Check sheet for the modelled part. Datum: model origin and axes. Units: mm. Face numbers are marked on the shaded views. A direction names the side the tool comes from. Round coordinates to 2 decimals unless told otherwise and drop trailing zeros. Write each loop counter-clockwise with the first axis right and the second up, starting at its lowest first coordinate (ties: lowest second). Pieces come first, ordered by that corner, then holes. Notation, with made-up numbers: (-14.75, 20) -> (27.25, 20) arc R33 ccw to (27.25, 57) -> close; hole circle Ø9 at (-25.5, 76.5). An arc over 180 degrees is marked (long way). One line per item, written item: value.
from build123d import *

# Parameters (mm, degrees)
SKETCH_1_R          = 1.25
SKETCH_1_R_2        = 1.5
EXTRUDE_1_DEPTH     = 0.5
SKETCH_2_W          = 9
SKETCH_2_H          = 0.5
EXTRUDE_2_DEPTH     = 5
CUT_EXTRUDE_1_REACH = 16.195
SKETCH_3_R          = 1


with BuildPart() as part:
    # 草图1 → 凸台-拉伸1 (new body)
    with BuildSketch(Plane.XY):
        with BuildLine():
            Line((0, 0), (9, 0))
            Line((9, 0), (6.667108595, 8.355095313))
            ThreePointArc((6.667108595, 8.355095313), (4.5, 10), (2.332891405, 8.355095313))
            Line((2.332891405, 8.355095313), (0, 0))
        make_face()
        with Locations((4.5, 7.75)):
            Circle(SKETCH_1_R, mode=Mode.SUBTRACT)
        with Locations((4.5, 3.5)):
            Circle(SKETCH_1_R_2, mode=Mode.SUBTRACT)
    extrude(amount=EXTRUDE_1_DEPTH)

    # 草图2 → 凸台-拉伸2 (add)
    with BuildSketch(Plane.XY.offset(0.5)):
        with Locations((4.5, 0.25)):
            Rectangle(SKETCH_2_W, SKETCH_2_H)
    extrude(amount=EXTRUDE_2_DEPTH)

    # 草图3 → 切除-拉伸1 (cut, up to next)
    with BuildSketch(Plane(origin=(0, 0.5, 0), x_dir=(1, 0, 0), z_dir=(0, 1, 0)), mode=Mode.PRIVATE) as cut_extrude_1_sk1:
        with Locations(Location((1.6, -3, 0), (0, 0, 270))):
            Circle(SKETCH_3_R)
    cut_extrude_1_tool1 = extrude(cut_extrude_1_sk1.sketch, amount=-CUT_EXTRUDE_1_REACH, mode=Mode.PRIVATE) & part.part
    # 草图3 → 切除-拉伸1 (cut, up to next)
    with BuildSketch(Plane(origin=(0, 0.5, 0), x_dir=(1, 0, 0), z_dir=(0, 1, 0)), mode=Mode.PRIVATE) as cut_extrude_1_sk2:
        with Locations(Location((7.4, -3, 0), (0, 0, 270))):
            Circle(SKETCH_3_R)
    cut_extrude_1_tool2 = extrude(cut_extrude_1_sk2.sketch, amount=-CUT_EXTRUDE_1_REACH, mode=Mode.PRIVATE) & part.part
    add(cut_extrude_1_tool1.solids().sort_by_distance((1.6, 0.5, 3))[0], mode=Mode.SUBTRACT)
    add(cut_extrude_1_tool2.solids().sort_by_distance((7.4, 0.5, 3))[0], mode=Mode.SUBTRACT)


solid = part.part
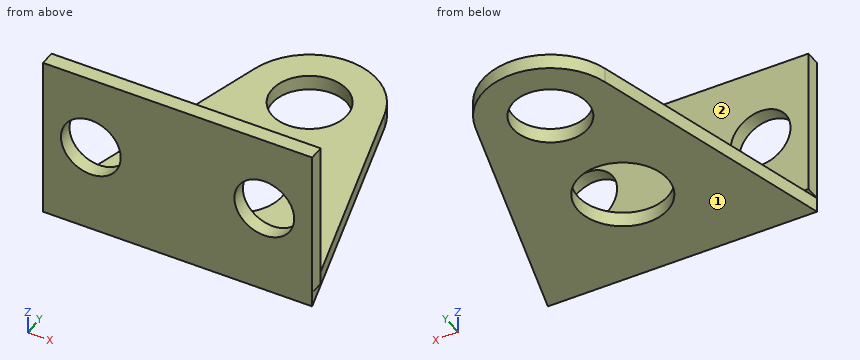
Item 1: Sectioned sample at D-D (x = 1.6). Enter the section's corners in (y, z).
Result set:
outline: (0, 0) -> (5.73, 0) -> (5.73, 0.5) -> (0.5, 0.5) -> (0.5, 2) -> (0, 2) -> close; (0, 4) -> (0.5, 4) -> (0.5, 5.5) -> (0, 5.5) -> close
Item 2: Depth check by flat-ended pin: pin 1 (1 mm diameter, centred on x = 4, z = 1, fed in from -Y); pin 2 (1.5 mm diameter, centred on x = 5, y = 5, fed in from +Z); pin 3 (3 mm diameter, centred on x = 6.5, z = 1.5, fed in from +Y). Enter the tip coordinate at first touch or a pass-through.
Result set:
pin 1: y = 0
pin 2: z = 0.5
pin 3: y = 9.82
Item 3: Sectioned sample at B-B (z = 3). Enter the section's corners in (x, y).
Result set:
outline: (0, 0) -> (0.6, 0) -> (0.6, 0.5) -> (0, 0.5) -> close; (2.6, 0) -> (6.4, 0) -> (6.4, 0.5) -> (2.6, 0.5) -> close; (8.4, 0) -> (9, 0) -> (9, 0.5) -> (8.4, 0.5) -> close
Item 4: Tool access check on the marked faces 1 and 2. Record the directions out of +Z, -Z, +X, -X, +Y, -Y that give a thin tool (end or side, any length) a straight path to the whole face; none if there is none.
Result set:
face 1: -Z, +X, -X, +Y, -Y
face 2: +Z, +X, -X, +Y
Item 5: Material ranges on line 1 along Y through (x, z) = (4.5, 0.2); line 2 along X through (y, z) = (0.25, 3); line 3 along Y through (x, z) = (6.5, 1.5), recorded low to high.
Result set:
line 1: 0 to 2, 5 to 6.5, 9 to 10
line 2: 0 to 0.6, 2.6 to 6.4, 8.4 to 9
line 3: 0 to 0.5
Item 6: Sectioned sample at A-A (y = 8). Enter the section's corners in (x, z), then the cut area to 3 significant figures.
Result set:
outline: (2.23, 0) -> (3.28, 0) -> (3.28, 0.5) -> (2.23, 0.5) -> close; (5.72, 0) -> (6.77, 0) -> (6.77, 0.5) -> (5.72, 0.5) -> close
area: 1.04 mm^2
Item 7: Sectioned sample at C-C (x = 3.5). Enter the section's corners in (y, z).
Result set:
outline: (0, 0) -> (2.38, 0) -> (2.38, 0.5) -> (0.5, 0.5) -> (0.5, 5.5) -> (0, 5.5) -> close; (4.62, 0) -> (7, 0) -> (7, 0.5) -> (4.62, 0.5) -> close; (8.5, 0) -> (9.77, 0) -> (9.77, 0.5) -> (8.5, 0.5) -> close
